Design review of the part built by this model. Coordinates are the model's own, in mm. A direction names the side the tool comes from. Give positions to 0.01 mm unless a question says otherwise; leave off trailing zeros. Loops run counter-clockwise (first coordinate to the right, second up) from the corner with the lowest first, then second, coordinate; pieces in that order, holes last.
from build123d import *

# Parameters (mm, degrees)
F1_DEPTH = 25.4
F2_R     = 3.175
F3_DEPTH = 34.925


with BuildPart() as f1:
    # F0 (on Top) → F1 (new body)
    with BuildSketch(Plane.XY):
        Polygon((3.175, 0), (0, 0), (0, -44.45), (34.925, -44.45), (34.925, 0), (31.75, 0), (31.75, -41.275), (3.175, -41.275), align=None)
    extrude(amount=F1_DEPTH)

    # F2 (on Right) → F3 (cut)
    with BuildSketch(Plane.YZ):
        with BuildLine():
            Line((0, 0), (0, 12.7))
            ThreePointArc((0, 12.7), (-3.719744, 3.719744), (-12.7, 0))
            Line((-12.7, 0), (0, 0))
        make_face()
        with BuildLine():
            ThreePointArc((-12.7, 25.4), (-3.719744, 21.680256), (0, 12.7))
            Line((0, 12.7), (0, 25.4))
            Line((0, 25.4), (-12.7, 25.4))
        make_face()
        with Locations((-12.7, 12.7)):
            Circle(F2_R)
    extrude(amount=F3_DEPTH, mode=Mode.SUBTRACT)


solid = f1.part
Q1. Wall thickness on line 1 (X direction, y = -40.5, z = 3) (3 decimals); line 2 (Y direction, x = 33.65, z = 12.7) (3 decimals); line 3 (Y direction, x = 17, z = 24) (3 decimals): over which ranges is each line inside the solid? List them lowest first.
Results:
line 1: x = 0 to 3.175, 31.75 to 34.925
line 2: y = -44.45 to -15.875, -9.525 to 0
line 3: y = -44.45 to -41.275
Q2. Draft analysis for pull direction Z (two halves, no side actions). For faces 1 (the face through (1.6, -11.2, 9.9)), 2 (the face through (16.09, -41.44, 0)), 3 (the face through (31.75, -20, 13)), state which applies: pulls with the +Z half, pulls with the -Z half, needs draft (parallel to the pull), parting line crosses it, or undercut.
Results:
face 1: undercut
face 2: pulls with the -Z half
face 3: needs draft
Q3. Take a section at B-B (z = 11.5). Give the number of separate pieces and of enclosed holes in the cut face, plus the area to 3 significant figures.
Results:
separate pieces: 3
enclosed holes: 0
area: 335 mm2
Q4. Take a section at C-C (z = 6.75). Give the boundary of the cut face in (x, y) (3 decimals), plus the area to 3 significant figures.
Results:
outline: (0, -44.45) - (34.925, -44.45) - (34.925, -1.48) - (31.75, -1.48) - (31.75, -41.275) - (3.175, -41.275) - (3.175, -1.48) - (0, -1.48) - close
area: 364 mm2
Q5. Tool access review of faces 4 (the face through (33.3, -11.2, 9.9)), 5 (the face through (3.175, -21, 13)): name each direction out of +Z, -Z, +X, -X, +Y, -Y from which nothing blocks a thin tool from reaching the whole face with its end or side.
Results:
face 4: +X, -X
face 5: +Z, -Z, +Y
Q6. Take a section at D-D (y = -4.5). Give the boundary of the cut face in (x, z) (3 decimals).
Results:
outline: (0, 3.002) - (3.175, 3.002) - (3.175, 22.398) - (0, 22.398) - close; (31.75, 3.002) - (34.925, 3.002) - (34.925, 22.398) - (31.75, 22.398) - close
Q7. Take a section at A-A (y = -31.5). Give the boundary of the cut face in (x, z) (3 decimals).
Results:
outline: (0, 0) - (3.175, 0) - (3.175, 25.4) - (0, 25.4) - close; (31.75, 0) - (34.925, 0) - (34.925, 25.4) - (31.75, 25.4) - close
Q8. Insertion check: pin 1 (6 mm diameter, centred on y = -18.5, z = 17.5, fed in from -X); pin 2 (12.5 mm diameter, centred on x = 12.5, z = 18.5, fed in from +Y) (3 decimals); pin 3 (3 mm diameter, centred on x = 23, y = -38.5, fed in from +Z). Each pin has a flat end and moves straight along its axis. Give the tip position at first contact, or say it passes through.
Results:
pin 1: stops at x = 0
pin 2: stops at y = -41.275
pin 3: passes through
